Design review of the part built by this model. Coordinates are the model's own, in mm. A direction names the side the tool comes from. Coordinates: 2 decimals unless noted, no trailing zeros.
Q1. Add section A-A, the plane z = -215. Give the number of separate pieces and of enclosed holes in the cut face, plus the area to 3 significant figures.
Q2. The part is to be moulded in two halves that separate along X. For faces 1 (the face through (284.099, 6, -215)), 2 (the face through (0, 6, -125)), 3 (the face through (352, 6, -254)), say which applies: +X half, -X half, draft (parallel to the pull), parting line (faces both ways), or undercut.
Q3. Clearance check with a flat-ended pin moving along its axis: pin 1 Ø1.5 at (x, y) = (278.5, 9) entering from -Z. State where the tip first meets the part, or that it passes through.
Q4. To check wall thickness, follow probe 1 along X at (y, z) = (10.5, -22) (3 decimals); probe 2 along Z at (x, y) = (524.5, 3.75). State the ranges of each line that lie inside material, in increasing order.
Q5. Machinability: for faces 4 (the face through (156, 6, -50.8)), 5 (the face through (371.704, 6, -216)), 6 (the face through (61, 6, -254)), which of the approach directions +Z, -Z, +X, -X, +Y, -Y give a long, thin tool a straight path to every point of the face, cutting with its end or side? Answer none if there is none.
from build123d import *

# Parameters (mm, degrees)
BOSS_EXTRUDE1_DEPTH = 12.7


with BuildPart() as part:
    # Sketch1 → Boss-Extrude1 (new body)
    with BuildSketch(Plane(origin=(0, 0, 0), x_dir=(1, 0, 0), z_dir=(0, 1, 0))):
        Polygon((0, 0), (0, 254), (31.75, 254), (31.75, 177.8), (41.275, 177.8), (41.275, 254), (80.3148, 254), (80.3148, 177.8), (89.8398, 177.8), (89.8398, 254), (128.8796, 254), (128.8796, 177.8), (138.4046, 177.8), (138.4046, 254), (177.4444, 254), (177.4444, 177.8), (186.9694, 177.8), (186.9694, 254), (226.0092, 254), (226.0092, 177.8), (235.5342, 177.8), (235.5342, 254), (274.574, 254), (274.574, 177.8), (284.099, 177.8), (284.099, 254), (323.1388, 254), (323.1388, 177.8), (332.6638, 177.8), (332.6638, 254), (371.7036, 254), (371.7036, 177.8), (381.2286, 177.8), (381.2286, 254), (420.2684, 254), (420.2684, 177.8), (429.7934, 177.8), (429.7934, 254), (468.8332, 254), (468.8332, 177.8), (478.3582, 177.8), (478.3582, 254), (517.398, 254), (517.398, 177.8), (527.05, 177.8), (527.05, 254), (558.8, 254), (558.8, 0), (409.575, 0), (409.575, 50.8), (396.875, 50.8), (396.875, 0), (161.925, 0), (161.925, 50.8), (149.225, 50.8), (149.225, 0), align=None)
    extrude(amount=BOSS_EXTRUDE1_DEPTH)


solid = part.part
Here are the results:
1. separate pieces: 12
1. enclosed holes: 0
1. area: 5,760 mm2
2. face 1: undercut
2. face 2: -X half
2. face 3: draft
3. pin 1: stops at z = -177.8
4. probe 1: x = 0 to 149.225, 161.925 to 396.875, 409.575 to 558.8
4. probe 2: z = -177.8 to 0
5. face 4: +Z, +Y, -Y
5. face 5: -Z, +Y, -Y
5. face 6: -Z, +X, -X, +Y, -Y
